Here's how the part is built. I have some questions about the finished solid (model axes, mm). Face numbers are marked on the shaded views. A direction names the side the tool comes from. Round coordinates to 2 decimals unless told otherwise and drop trailing zeros. Order: outer loops, then holes, each group sorted by start corner. A loop starts at its lowest first (then second) coordinate and runs counter-clockwise, first axis right, second up. Notation, with made-up numbers: (66.25, 80.25) - (103.25, 80.25) arc R12 cw to (103.25, 102.25) - close; hole circle Ø3 at (-17.75, 41.25). An arc over 180 degrees is marked (long way). Answer as a JSON object with one key per item and string values.
Autodesk Inventor part; units mm, degrees
ref_plane "YZ Plane" through (0, 0, 0) normal (1, 0, 0) x (0, 1, 0)
ref_plane "XZ Plane" through (0, 0, 0) normal (0, 1, 0) x (-1, 0, 0)
ref_plane "XY Plane" through (0, 0, 0) normal (0, 0, 1) x (1, 0, 0)
sketch "スケッチ1" plane through (0, 0, 0) normal (0, 0, 1) x (1, 0, 0)
  circle A0 centre (0, 0) radius 7.25
  dimension "d0" = 14.5
extrude "押し出し1" add sketch "スケッチ1" along normal blind 48.8
sketch "スケッチ2" plane through (0, 0, 48.8) normal (0, 0, 1) x (1, 0, 0)
  circle A0 centre (0, 0) radius 2.5
  dimension "d3" = 5
extrude "押し出し2" add sketch "スケッチ2" along normal blind 1.7
fillet "フィレット1" radius 0.25 4 edges at (-7.25, 0, 48.8) (-7.25, 0, 0) (-2.5, 0, 50.5) (-2.5, 0, 48.8)
properties part number "battery"
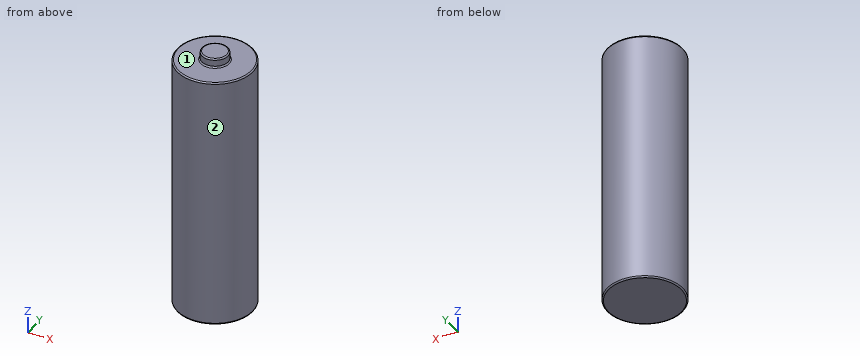
1. Imagine slicing it at A-A (y = 0). List the corners of the cut face in (x, z) for me.
Responses:
{"outline": "(-7.25, 0.25) arc R0.25 ccw to (-7, 0) - (7, 0) arc R0.25 ccw to (7.25, 0.25) - (7.25, 48.55) arc R0.25 ccw to (7, 48.8) - (2.75, 48.8) arc R0.25 cw to (2.5, 49.05) - (2.5, 50.25) arc R0.25 ccw to (2.25, 50.5) - (-2.25, 50.5) arc R0.25 ccw to (-2.5, 50.25) - (-2.5, 49.05) arc R0.25 cw to (-2.75, 48.8) - (-7, 48.8) arc R0.25 ccw to (-7.25, 48.55) - close"}
2. Imagine slicing it at C-C (z = 16.5). List the corners of the cut face in (x, y) for me.
Responses:
{"outline": "circle Ø14.5 at (0, 0)"}
3. For the marked faces 1 and 2, which set-ups out of +Z, -Z, +X, -X, +Y, -Y let a thin tool reach every point of the face, with its end or its side?
Responses:
{"face 1": "+Z", "face 2": "+Z, -Z"}
4. If I drill on L1, parallel to Z at x = -2.75, y = -2; L2, parallel to Y at x = -0.25, z = 42.5; L3, parallel to X at y = -1.75, z = 11.5, over which ranges is the centre line in solid material (lowest first)? Write a range as [from, to].
Responses:
{"L1": "[0, 48.8]", "L2": "[-7.25, 7.25]", "L3": "[-7.04, 7.04]"}
5. For P1, Ø2, axis at x = -2.5, z = 15.5, coming from the -Y side; P2, Ø1.5, axis at x = 4.5, z = 22, coming from the -Y side; P3, Ø5, axis at y = -2.5, z = 8, coming from the -X side; P4, Ø4, axis at y = -5.5, z = 5.5, coming from the -X side, each with a flat end and sliding along its axis, tell me the tip position at first contact or that it passes through.
Responses:
{"P1": "y = -7.09", "P2": "y = -6.2", "P3": "x = -7.25", "P4": "x = -6.35"}
